Input: dimensioned drawing with shaded views. Units: mm. Origin: part minimum x, y, z. A direction names the side the tool comes from. Coordinates: 2 decimals unless noted, no trailing zeros. Order: outer loops, then holes, each group sorted by start corner. A loop starts at its lowest first (then second) coordinate and runs counter-clockwise, first axis right, second up. Notation, with made-up numbers: (31, 14.25) -> (77, 14.25) arc R25 cw to (77, 51.25) -> close; hole circle Ø8 at (-13, 50). An arc over 180 degrees is marked (long way). Write item = value, one per line. Start each with the question number.
Item 1: Section query C-C (x = 2.1). Output: boundary loops of the cut face in (y, z).
Item 2: Contact query for a flat-ended pin moving along its axis: pin 1 (3 mm diameter, centred on y = 6.5, z = 0.5, fed in from -X). Output: stop coordinate, or through.
Item 3: Mould query, pull axis X, two halves, no side actions, for the marked faces 3, 4 and 5. Classes: released by +X, released by -X, zero draft, split by the parting line, or undercut.
Item 4: Section query A-A (z = 1.4). Output: boundary loops of the cut face in (x, y).
Item 5: Set-up query: the marked faces 1 and 2. Return all of +Z, -Z, +X, -X, +Y, -Y with unobstructed straight access to the full face (end or side cutting, diameter ignored); none if empty.
Item 6: Ray query, line 1 along X through (y, z) = (2.75, 1.1); line 2 along Z through (x, y) = (3.1, 2.5). Return the intervals inside material, ascending. Write a range as [from, to].
Item 7: Section query B-B (y = 4). Output: boundary loops of the cut face in (x, z), then the cut area to 3 significant figures.
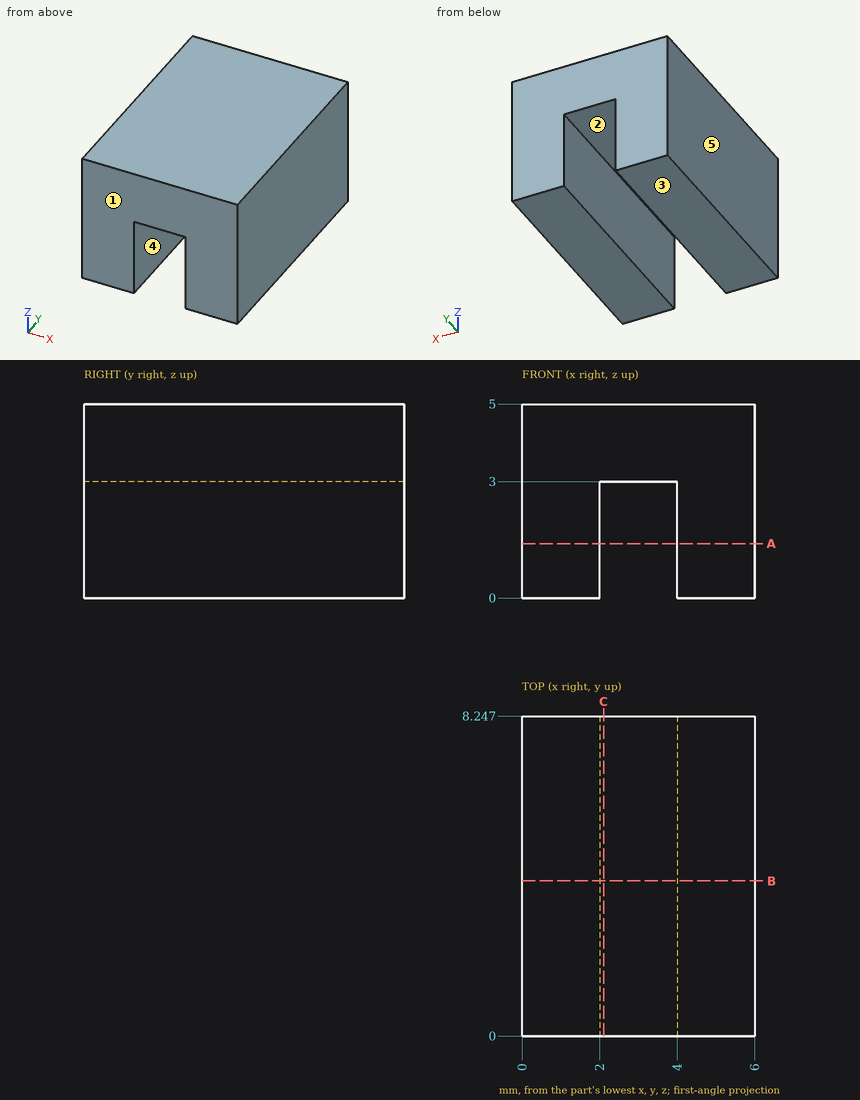
Computed:
q1.outline = (0, 3) -> (8.25, 3) -> (8.25, 5) -> (0, 5) -> close
q2.pin_1 = 0
q3.face_3 = zero draft
q3.face_4 = undercut
q3.face_5 = released by -X
q4.outline = (0, 0) -> (2, 0) -> (2, 8.25) -> (0, 8.25) -> close; (4, 0) -> (6, 0) -> (6, 8.25) -> (4, 8.25) -> close
q5.face_1 = +Z, -Z, +X, -X, -Y
q5.face_2 = -Z, +Y, -Y
q6.line_1 = [0, 2], [4, 6]
q6.line_2 = [3, 5]
q7.outline = (0, 0) -> (2, 0) -> (2, 3) -> (4, 3) -> (4, 0) -> (6, 0) -> (6, 5) -> (0, 5) -> close
q7.area = 24.0 mm^2
